Check sheet for the drawn part. Datum: minimum x, y, z corner. Units: mm. Coordinates: 2 decimals unless noted, no trailing zeros. Order: outer loops, then holes, each group sorted by start corner. A loop starts at its lowest first (then second) coordinate and runs counter-clockwise, first axis right, second up.
1. Cross-section at B-B (x = 40.5). Enter the section's corners in (y, z) (3 decimals).
2. Thickness scan on line 1 (Z direction, x = 25.4, y = 2); line 2 (X direction, y = 7.25, z = 247.65); line 3 (Z direction, x = 46.5, y = 7.25). Record the ranges inside material, lowest first.
3. Gauge pin test, flat ends, axial feed: pin 1 Ø3 at (x, y) = (25, 5.5) entering from +Z; pin 2 Ø15 at (x, z) = (27, 900.5) entering from -Y (3 decimals). Record the tip position at first contact, or that the pin passes through.
4. Cross-section at A-A (y = 6.5). Count the separate pieces of the cut face and the enclosed holes in it, then the cut area to 3 significant figures.
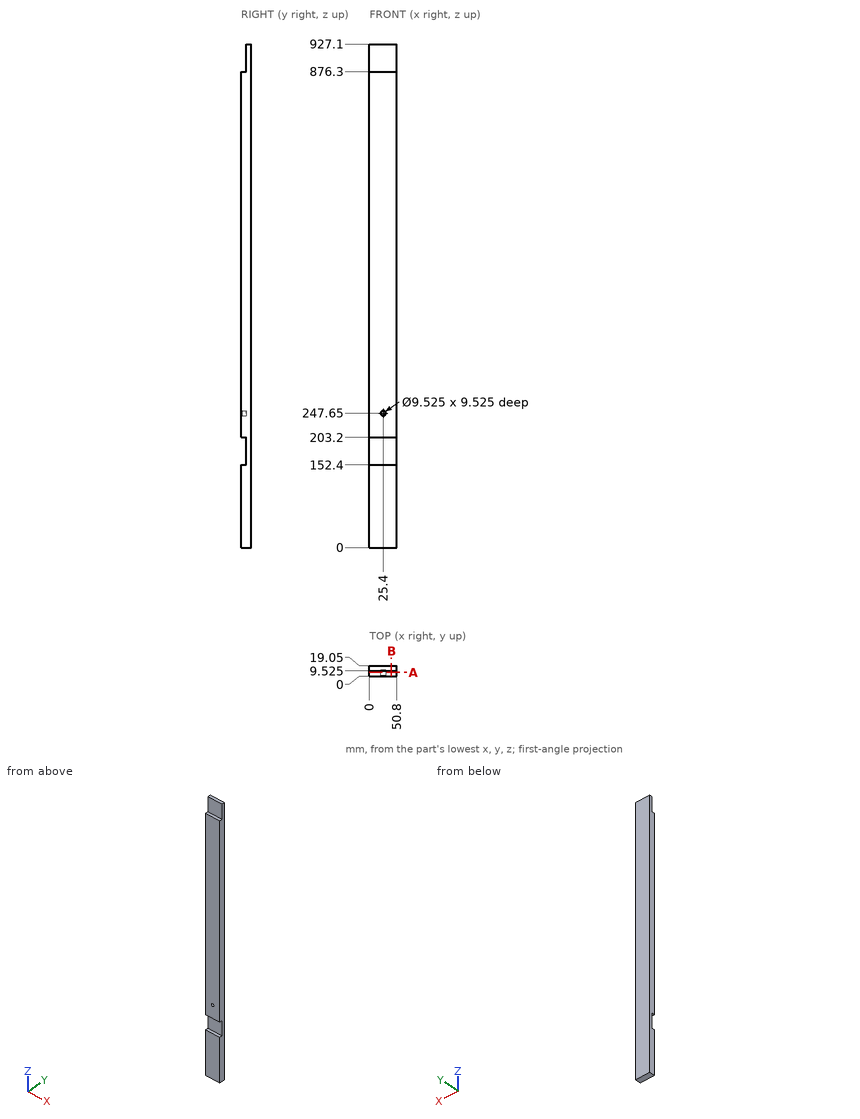
Data:
1. outline: (0, 0) - (19.05, 0) - (19.05, 927.1) - (9.525, 927.1) - (9.525, 876.3) - (0, 876.3) - (0, 203.2) - (9.525, 203.2) - (9.525, 152.4) - (0, 152.4) - close
2. line 1: z = 0 to 152.4, 203.2 to 242.89, 252.41 to 876.3
2. line 2: x = 0 to 20.64, 30.16 to 50.8
2. line 3: z = 0 to 152.4, 203.2 to 876.3
3. pin 1: stops at z = 876.3
3. pin 2: stops at y = 9.525
4. separate pieces: 2
4. enclosed holes: 1
4. area: 41,900 mm2
